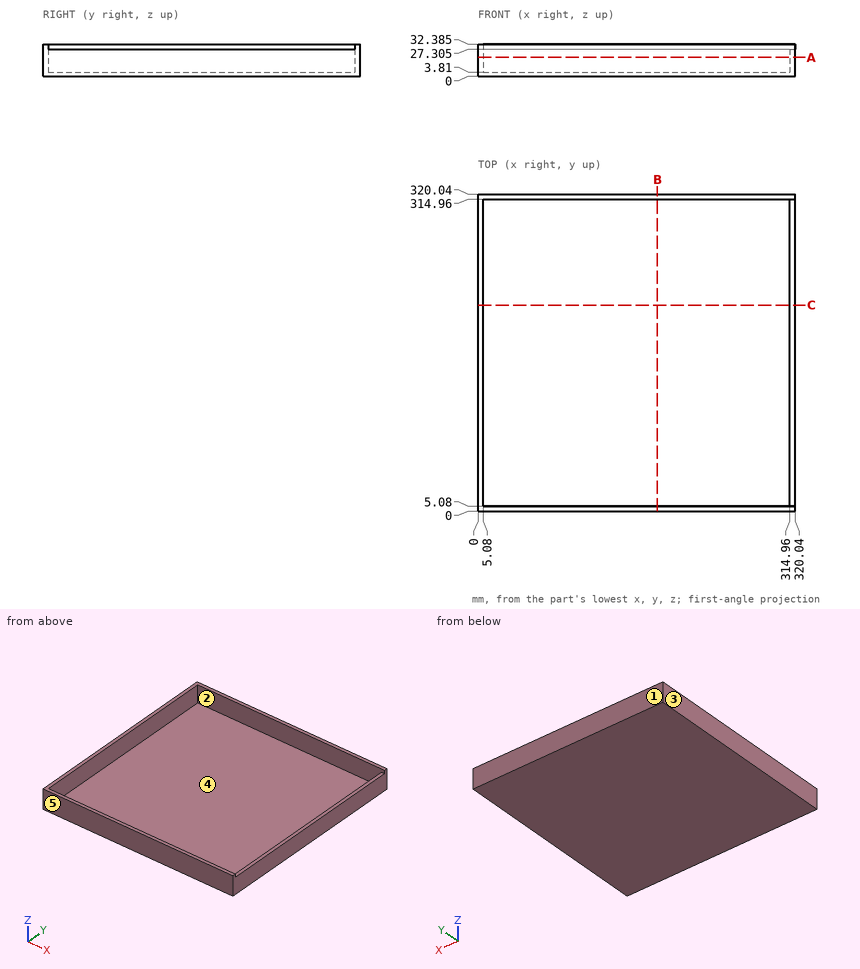
Input: dimensioned drawing with shaded views. Units: mm. Origin: part minimum x, y, z. A direction names the side the tool comes from. Coordinates: 2 decimals unless noted, no trailing zeros. Loops run counter-clockwise (first coordinate to the right, second up) from the corner with the lowest first, then second, coordinate; pieces in that order, holes last. Notation, with made-up numbers: M -27.75,-23.5 L 5.25,-23.5 A19 cw 5.25,6.5 Z; hole C -14.75,-14 d11. An arc over 180 degrees is marked long. Put each result on its own line as item: value.
(1) Cut plane C-C on y = 208. Return the cut outline in (x, z) (3 decimals).
Answer sheet:
outline: M 0,0 L 320.04,0 L 320.04,27.305 L 314.96,27.305 L 314.96,3.81 L 5.08,3.81 L 5.08,32.385 L 0,32.385 Z
(2) First-contact query: pin 1 (5.5 mm diameter, centred on x = 317, y = 207.5, fed in from +Z) (3 decimals); pin 2 (6 mm diameter, centred on x = 104, y = 267.5, fed in from +Z). Flat tips, straight axial feed; report the tip coordinate or a pass-through.
Answer sheet:
pin 1: stops at z = 27.305
pin 2: stops at z = 3.81
(3) Access query for the marked faces 1 and 2. Directions: +Z, -Z, +X, -X, +Y, -Y. A direction counts if a zero-diameter tool reaches every point of the face in a straight line with its end or side. Return the directions, or none.
Answer sheet:
face 1: +Z, -Z, +X, -X, +Y
face 2: +Z
(4) Cut plane B-B on x = 181. Return the cut outline in (y, z) (3 decimals).
Answer sheet:
outline: M 0,0 L 320.04,0 L 320.04,32.385 L 314.96,32.385 L 314.96,3.81 L 5.08,3.81 L 5.08,32.385 L 0,32.385 Z
(5) Draft query along Y for the marked faces 3, 4 and 5. Return one class per face: pulls with the +Y half, pulls with the -Y half, needs draft (parallel to the pull), parting line crosses it, or undercut.
Answer sheet:
face 3: needs draft
face 4: undercut
face 5: pulls with the -Y half
(6) Cut plane A-A on z = 19. Return the cut outline in (x, y).
Answer sheet:
outline: M 0,0 L 320.04,0 L 320.04,320.04 L 0,320.04 Z; hole M 5.08,5.08 L 314.96,5.08 L 314.96,314.96 L 5.08,314.96 Z
(7) Material intervals for probe 1 along Y at (x, z) = (43, 29.5); probe 2 along Z at (x, y) = (44, 123), sorted ascending.
Answer sheet:
probe 1: y = 0 to 5.08, 314.96 to 320.04
probe 2: z = 0 to 3.81
